```python
from build123d import *

# Parameters (mm, degrees)
SKETCH_1_R      = 120
EXTRUDE_1_DEPTH = 5
MM_2_D          = 8
MM_2_DEPTH      = 20
MM_2_TIP        = 2.403442476
SKETCH_6_R      = 30
SKETCH_6_R_2    = 20
EXTRUDE_2_DEPTH = 200


with BuildPart() as part:
    # 草图1 → 凸台-拉伸1 (new body)
    with BuildSketch(Plane(origin=(0, 0, 0), x_dir=(1, 0, 0), z_dir=(0, 1, 0))):
        with Locations(Location((0, 0, 0), (0, 0, 270))):
            Circle(SKETCH_1_R)
    extrude(amount=EXTRUDE_1_DEPTH)

    # 大小mm 暗销孔2
    with Locations(Plane(origin=(0, 5, -60), x_dir=(0, 0, 1), z_dir=(0, 1, 0))):
        with Locations((0, 0), (60, -60), (120, 0), (60, 60)):
            Hole(MM_2_D / 2, depth=MM_2_DEPTH)
            with Locations((0, 0, -(MM_2_DEPTH + MM_2_TIP / 2))):  # 118° drill point
                Cone(0, MM_2_D / 2, MM_2_TIP, mode=Mode.SUBTRACT)

    # 草图6 → 凸台-拉伸2 (add)
    with BuildSketch(Plane(origin=(0, 5, 0), x_dir=(1, 0, 0), z_dir=(0, 1, 0))):
        with Locations(Location((0, 0, 0), (0, 0, 270))):
            Circle(SKETCH_6_R)
        with Locations(Location((0, 0, 0), (0, 0, 270))):
            Circle(SKETCH_6_R_2, mode=Mode.SUBTRACT)
    extrude(amount=EXTRUDE_2_DEPTH)


solid = part.part
```
Input: part model. Units: mm. Frame: model coordinates. A direction names the side the tool comes from. Round coordinates to 2 decimals unless told otherwise and drop trailing zeros. Write each loop counter-clockwise with the first axis right and the second up, starting at its lowest first coordinate (ties: lowest second). Pieces come first, ordered by that corner, then holes. Notation, with made-up numbers: (-22, 52) -> (1, 52) arc R10 cw to (1, 66) -> close; hole circle Ø2 at (-28.5, -26). An arc over 180 degrees is marked (long way). Answer as CSV lines item,"result".
1. Section C-C (y = 64). Return the cut outline in (x, z).
Geometry says:
outline,"circle Ø60 at (0, 0); hole circle Ø40 at (0, 0)"
2. Section A-A (x = 0). Return the cut outline in (y, z), plus the area to 3 significant figures.
Geometry says:
outline,"(0, -120) -> (5, -120) -> (5, -64) -> (0, -64) -> close; (0, -56) -> (5, -56) -> (5, -30) -> (205, -30) -> (205, -20) -> (5, -20) -> (5, 20) -> (205, 20) -> (205, 30) -> (5, 30) -> (5, 56) -> (0, 56) -> close; (0, 64) -> (5, 64) -> (5, 120) -> (0, 120) -> close"
area,"5,120 mm^2"
3. Reachability of faces 1 (the cylindrical face through (-19.524, 103.6, -4.336)), 2 (the cylindrical face through (5.276, 2.465, -119.884)) from +Z, -Z, +X, -X, +Y, -Y: full face, straight path, thin tool, end or side. Return the list, or none.
Geometry says:
face 1,"+Y"
face 2,"+Y, -Y"
4. Section B-B (z = 0). Return the cut outline in (x, y).
Geometry says:
outline,"(-120, 0) -> (-64, 0) -> (-64, 5) -> (-120, 5) -> close; (-56, 0) -> (56, 0) -> (56, 5) -> (30, 5) -> (30, 205) -> (20, 205) -> (20, 5) -> (-20, 5) -> (-20, 205) -> (-30, 205) -> (-30, 5) -> (-56, 5) -> close; (64, 0) -> (120, 0) -> (120, 5) -> (64, 5) -> close"
5. Mould query, pull axis X, two halves, no side actions, for faces 3 (the cylindrical face through (1.201, 2.465, 56.185)), 4 (the flat face through (-20, 205, 6)), 5 (the cylindrical face through (1.32, 103.6, -29.97)), 6 (the cylindrical face through (1.201, 2.465, -63.815)). Classes: +X half, -X half, draft (parallel to the pull), parting line (faces both ways), or undercut.
Geometry says:
face 3,"undercut"
face 4,"draft"
face 5,"parting line"
face 6,"undercut"
6. Section D-D (z = 60). Return the cut outline in (x, y).
Geometry says:
outline,"(-103.92, 0) -> (-4, 0) -> (-4, 5) -> (-103.92, 5) -> close; (4, 0) -> (103.92, 0) -> (103.92, 5) -> (4, 5) -> close"
7. Contact query for flat-ended pins moving along their axis: P1, Ø5, axis at x = 0, z = -60, coming from the +Y side; P2, Ø10.5, axis at x = 60, z = 0, coming from the +Y side; P3, Ø4, axis at x = -14.5, y = 33.5, coming from the -Z side; P4, Ø1, axis at x = 21, y = 183.5, coming from the +Z side. Output: stop coordinate, or through.
Geometry says:
P1,"passes through"
P2,"stops at y = 5"
P3,"stops at z = -27.27"
P4,"stops at z = 21.9"
8. Ray query, L1, parallel to X at y = 3.05, z = 0; L2, parallel to Y at x = -50.5, z = -58.5; L3, parallel to Z at x = -11, y = 97.5. Return the intervals inside material, ascending. Write a range as [from, to].
Geometry says:
L1,"x = [-120, -64], [-56, 56], [64, 120]"
L2,"y = [0, 5]"
L3,"z = [-27.91, -16.7], [16.7, 27.91]"
